from build123d import *

# Parameters (mm, degrees)
SKETCH1_R           = 1.5
BOSS_EXTRUDE1_DEPTH = 2


with BuildPart() as part:
    # Sketch1 → Boss-Extrude1 (new body)
    with BuildSketch(Plane(origin=(0, 0, 0), x_dir=(1, 0, 0), z_dir=(0, 1, 0))):
        Polygon((0, 0), (2, 0), (2, 5), (4, 5), (4, 0), (10, 0), (10, 5), (12, 5), (12, 0), (72.4, 0), (72.4, 5), (74.4, 5), (74.4, 0), (80.4, 0), (80.4, 5), (82.4, 5), (82.4, 0), (84.4, 0), (84.4, 45), (82.4, 45), (82.4, 40), (80.4, 40), (80.4, 45), (74.4, 45), (74.4, 40), (72.4, 40), (72.4, 45), (12, 45), (12, 40), (10, 40), (10, 45), (4, 45), (4, 40), (2, 40), (2, 45), (0, 45), align=None)
        with Locations(Location((7, 42.5, 0), (0, 0, 270))):
            Circle(SKETCH1_R, mode=Mode.SUBTRACT)
        with Locations(Location((77.4, 42.5, 0), (0, 0, 90))):
            Circle(SKETCH1_R, mode=Mode.SUBTRACT)
        with Locations(Location((7, 2.5, 0), (0, 0, 90))):
            Circle(SKETCH1_R, mode=Mode.SUBTRACT)
        with Locations(Location((77.4, 2.5, 0), (0, 0, 270))):
            Circle(SKETCH1_R, mode=Mode.SUBTRACT)
    extrude(amount=BOSS_EXTRUDE1_DEPTH)


solid = part.part
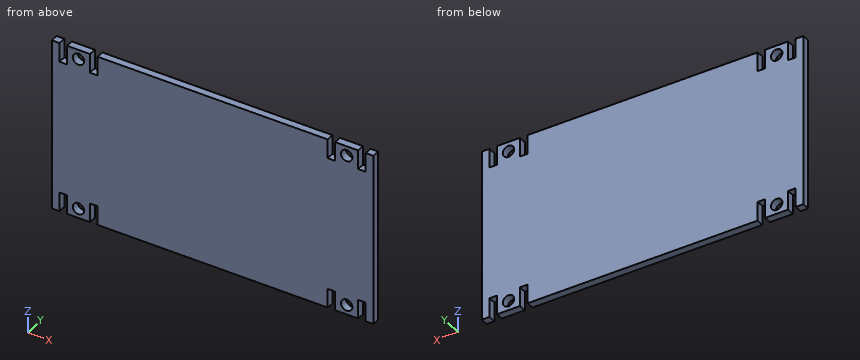
Read the model definition and answer for the solid it produces. Units are mm, in the model's axes. Round coordinates to 2 decimals unless told otherwise and drop trailing zeros. Loops run counter-clockwise (first coordinate to the right, second up) from the corner with the lowest first, then second, coordinate; pieces in that order, holes last.
Q1. Section A-A on x = 7 is taken. Write down the section's boundary in (y, z).
Q2. Consider probe 1 along X at (y, z) = (0.5, -4.5); probe 2 along Z at (x, y) = (77.4, 1.55). Determine where each line is inside the solid, lowest interval first.
Q3. Each of these flat-tipped pins is pushed along its axis until it touches: pin 1 (0.6 mm diameter, centred on x = 81.5, y = 0.5, fed in from -Z); pin 2 (0.6 mm diameter, centred on x = 11, y = 1.5, fed in from +Z). Where does it stop, or does it pass through?
Q4. Section C-C on y = 0.75 is taken. Give the number of separate pieces and of enclosed holes in the cut face, and give its area (3 significant figures).
Q5. Section B-B on z = -42.5 is taken. Write down the section's boundary in (x, y).
Output:
1. outline: (0, -45) - (2, -45) - (2, -44) - (0, -44) - close; (0, -41) - (2, -41) - (2, -4) - (0, -4) - close; (0, -1) - (2, -1) - (2, 0) - (0, 0) - close
2. probe 1: x = 0 to 2, 4 to 10, 12 to 72.4, 74.4 to 80.4, 82.4 to 84.4
2. probe 2: z = -45 to -44, -41 to -4, -1 to 0
3. pin 1: stops at z = -40
3. pin 2: stops at z = -5
4. separate pieces: 1
4. enclosed holes: 4
4. area: 3,690 mm2
5. outline: (0, 0) - (2, 0) - (2, 2) - (0, 2) - close; (4, 0) - (5.5, 0) - (5.5, 2) - (4, 2) - close; (8.5, 0) - (10, 0) - (10, 2) - (8.5, 2) - close; (12, 0) - (72.4, 0) - (72.4, 2) - (12, 2) - close; (74.4, 0) - (75.9, 0) - (75.9, 2) - (74.4, 2) - close; (78.9, 0) - (80.4, 0) - (80.4, 2) - (78.9, 2) - close; (82.4, 0) - (84.4, 0) - (84.4, 2) - (82.4, 2) - close
